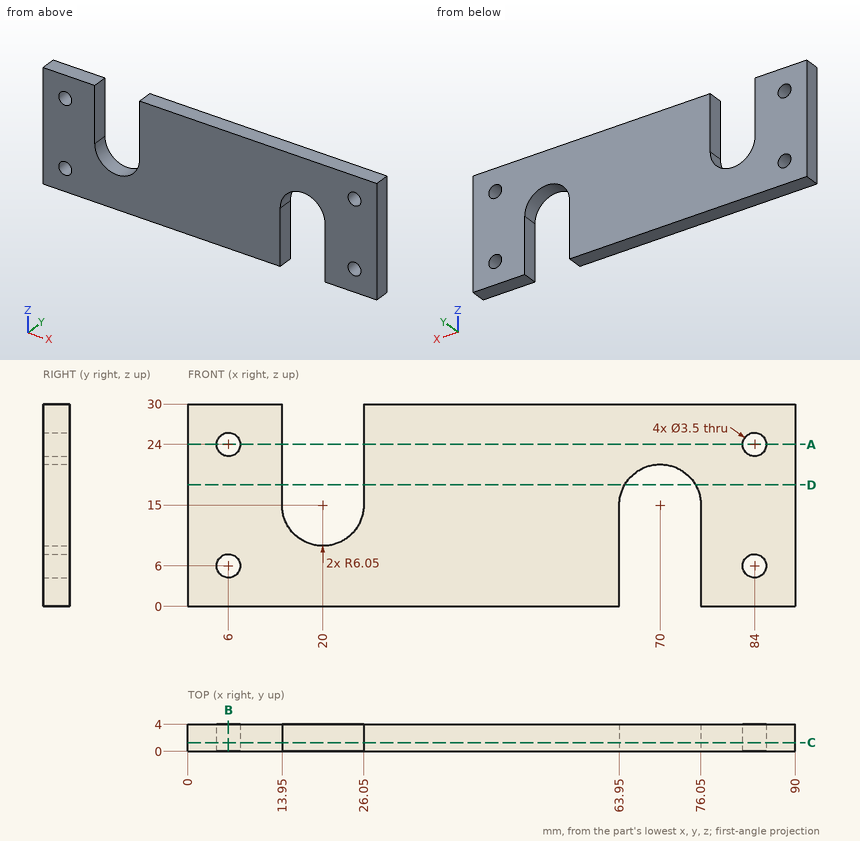
Verification items for this drawing (mm, ordinates from the low corner). Coordinates: 2 decimals unless noted, no trailing zeros. Order: outer loops, then holes, each group sorted by start corner. A loop starts at its lowest first (then second) coordinate and runs counter-clockwise, first axis right, second up. Notation, with made-up numbers: M 65,22 L 102,22 A11 cw 102,31 Z; hole C 5,-8 d1. An arc over 180 degrees is marked long. One line per item, written item: value. Start each with the question number.
Item 1: Depth check by flat-ended pin: P1, Ø3, axis at x = 6, z = 6, coming from the +Y side. Enter the tip coordinate at first touch or a pass-through.
Item 2: Sectioned sample at C-C on y = 1.3. Record the cut outline in (x, z), then the cut area to 3 significant figures.
Item 3: Sectioned sample at D-D on z = 18. Record the cut outline in (x, y), then the cut area to 3 significant figures.
Item 4: Sectioned sample at B-B on x = 6. Record the cut outline in (y, z), then the cut area to 3 significant figures.
Item 5: Thickness scan on probe 1 along X at (y, z) = (3.05, 24); probe 2 along Z at (x, y) = (6, 2.5); probe 3 along X at (y, z) = (2.8, 6). Record the ranges inside material, lowest first.
Item 6: Sectioned sample at A-A on z = 24. Record the cut outline in (x, y), then the cut area to 3 significant figures.
Calculated:
1. P1: through
2. outline: M 0,0 L 63.95,0 L 63.95,15 A6.05 cw 76.05,15 L 76.05,0 L 90,0 L 90,30 L 26.05,30 L 26.05,15 A6.05 cw 13.95,15 L 13.95,30 L 0,30 Z; hole C 6,6 d3.5; hole C 6,24 d3.5; hole C 84,6 d3.5; hole C 84,24 d3.5
2. area: 2,180 mm^2
3. outline: M 0,0 L 13.95,0 L 13.95,4 L 0,4 Z; M 26.05,0 L 64.75,0 L 64.75,4 L 26.05,4 Z; M 75.25,0 L 90,0 L 90,4 L 75.25,4 Z
3. area: 270 mm^2
4. outline: M 0,0 L 4,0 L 4,4.25 L 0,4.25 Z; M 0,7.75 L 4,7.75 L 4,22.25 L 0,22.25 Z; M 0,25.75 L 4,25.75 L 4,30 L 0,30 Z
4. area: 92.0 mm^2
5. probe 1: 0 to 4.25, 7.75 to 13.95, 26.05 to 82.25, 85.75 to 90
5. probe 2: 0 to 4.25, 7.75 to 22.25, 25.75 to 30
5. probe 3: 0 to 4.25, 7.75 to 63.95, 76.05 to 82.25, 85.75 to 90
6. outline: M 0,0 L 4.25,0 L 4.25,4 L 0,4 Z; M 7.75,0 L 13.95,0 L 13.95,4 L 7.75,4 Z; M 26.05,0 L 82.25,0 L 82.25,4 L 26.05,4 Z; M 85.75,0 L 90,0 L 90,4 L 85.75,4 Z
6. area: 284 mm^2
